Work out the finished part from the listing and answer in its coordinate system (mm). Round coordinates to 2 decimals unless told otherwise and drop trailing zeros. Order: outer loops, then holes, each group sorted by start corner. A loop starts at its lowest first (then second) coordinate and runs counter-clockwise, first axis right, second up. Notation, with made-up numbers: (40, 49) -> (63, 49) arc R23 cw to (63, 76) -> close; hole circle Ø11 at (-5.75, 84.5). An arc over 180 degrees is marked (long way). Use a Markdown table: item, result. Add a question column.
Item 1: For a pull along X with two mould halves and no side action, classify faces 1 (the cylindrical face through (25.68, 2.47, -0.25)), 2 (the flat face through (-25.128, 2, 22)), 3 (the flat face through (3, 5, 19)), 4 (the flat face through (29.337, 2.535, -8.867)) as +X half, -X half, draft (parallel to the pull), parting line (faces both ways), or undercut.
Item 2: Find the intervals of material crossed by L1, parallel to Z at x = -21.5, y = 3.55; L2, parallel to X at y = 0.35, z = -1.5; L3, parallel to Z at x = -23, y = 1.6, in increasing order. Write a range as [from, to].
Item 3: A cutting plane is placed at B-B, the plane y = 3.9. Determine the outline of the cut face in (x, z).
Item 4: A cutting plane is placed at A-A, the plane z = -2.5. Determine the outline of the cut face in (x, y), plus the area to 3 significant figures.
from build123d import *

# Parameters (mm, degrees)
SKETCH1_W           = 57
SKETCH1_H           = 62.1
SKETCH1_W_2         = 42
SKETCH1_H_2         = 49.6
BOSS_EXTRUDE1_DEPTH = 5
SKETCH2_W           = 42
SKETCH2_H           = 49.6
BOSS_EXTRUDE2_DEPTH = 5
M6_TAPPED_HOLE1_D   = 5
CUT_EXTRUDE1_DEPTH  = 5


with BuildPart() as part:
    # Sketch1 → Boss-Extrude1 (new body)
    with BuildSketch(Plane(origin=(0, 0, 0), x_dir=(1, 0, 0), z_dir=(0, 1, 0))):
        with Locations((3.372056515, -19.15989011)):
            Rectangle(SKETCH1_W, SKETCH1_H)
        with Locations((3.372056515, -17.90989011)):
            Rectangle(SKETCH1_W_2, SKETCH1_H_2, mode=Mode.SUBTRACT)
    extrude(amount=BOSS_EXTRUDE1_DEPTH)

    # Sketch2 → Boss-Extrude2 (add)
    with BuildSketch(Plane.XZ):
        with Locations((3.372056515, 17.90989011)):
            Rectangle(SKETCH2_W, SKETCH2_H)
    extrude(amount=-BOSS_EXTRUDE2_DEPTH)

    # M6 Tapped Hole1 (through all)
    with Locations(Plane(origin=(-21.377943485, 5, -0.79010989), x_dir=(0, 0, 1), z_dir=(0, 1, 0))):
        with Locations((0, 0), (45, 0), (45, 49.5), (0, 49.5)):
            Hole(M6_TAPPED_HOLE1_D / 2)

    # Sketch9 → Cut-Extrude1 (cut)
    with BuildSketch(Plane(origin=(0, 5, 0), x_dir=(1, 0, 0), z_dir=(0, 1, 0))):
        Polygon((-25.127943485, 11.89010989), (-25.127943485, 6.89010989), (-20.128034648, 10.790006378), (26.871965352, 10.790148591), (31.872056515, 6.89010989), (31.872056515, 11.89010989), align=None)
    extrude(amount=-CUT_EXTRUDE1_DEPTH, mode=Mode.SUBTRACT)


solid = part.part
Reported:
| question | item | result |
|---|---|---|
| 1 | face 1 | undercut |
| 1 | face 2 | -X half |
| 1 | face 3 | draft |
| 1 | face 4 | +X half |
| 2 | L1 | [-9.72, -3.29], [1.71, 41.71], [46.71, 50.21] |
| 2 | L2 | [-25.13, -23.78], [-18.98, 25.72], [30.52, 31.87] |
| 2 | L3 | [-8.55, -2.69], [1.11, 42.31], [46.11, 50.21] |
| 3 | outline | (-25.13, -6.89) -> (-20.13, -10.79) -> (26.87, -10.79) -> (31.87, -6.89) -> (31.87, 50.21) -> (-25.13, 50.21) -> close; hole circle Ø5 at (-21.38, -0.79); hole circle Ø5 at (-21.38, 44.21); hole circle Ø5 at (28.12, -0.79); hole circle Ø5 at (28.12, 44.21) |
| 4 | outline | (-25.13, 0) -> (-23.2, 0) -> (-23.2, 5) -> (-25.13, 5) -> close; (-19.55, 0) -> (26.3, 0) -> (26.3, 5) -> (-19.55, 5) -> close; (29.95, 0) -> (31.87, 0) -> (31.87, 5) -> (29.95, 5) -> close |
| 4 | area | 249 mm² |
